Job drawing, mm, ordinate dimensions from the low corner. One solid piece. Give positions to 0.01 mm unless a question says otherwise; leave off trailing zeros. Order: outer loops, then holes, each group sorted by start corner. A loop starts at its lowest first (then second) coordinate and runs counter-clockwise, first axis right, second up. Notation, with made-up numbers: (7.5, 33.5) - (64.5, 33.5) arc R30 ccw to (64.5, 68.5) - close; hole circle Ø4 at (75.5, 39.25). An arc over 180 degrees is marked (long way). Write each question's results on one line, items separated by ' | '. Start each with the question number.
1) Cut at A-A on z = 301.5. List the corners of the cut face in (x, y).
2) Drop flat-ended pins along their axis: pin 1 Ø5 at (x, y) = (211, 175.5) entering from +Z (1 decimal); pin 2 Ø6 at (x, y) = (96, 358.5) entering from +Z; pin 3 Ø10 at (x, y) = (312.5, 371.5) entering from +Z. Give the stop position or say it passes through.
3) Cut at C-C on y = 450.5. List the corners of the cut face in (x, z), plus the area to 3 significant figures.
4) Drill centre lines: line 1 along X through (y, z) = (59, 75); line 2 along Y through (x, z) = (479, 47); line 3 along Z through (x, y) = (347, 65). Where is each one in solid material? Low to high. Write a range as from..to.
5) Cut at B-B on x = 260. List the corners of the cut face in (y, z) (1 decimal), plus the area to 3 significant figures.
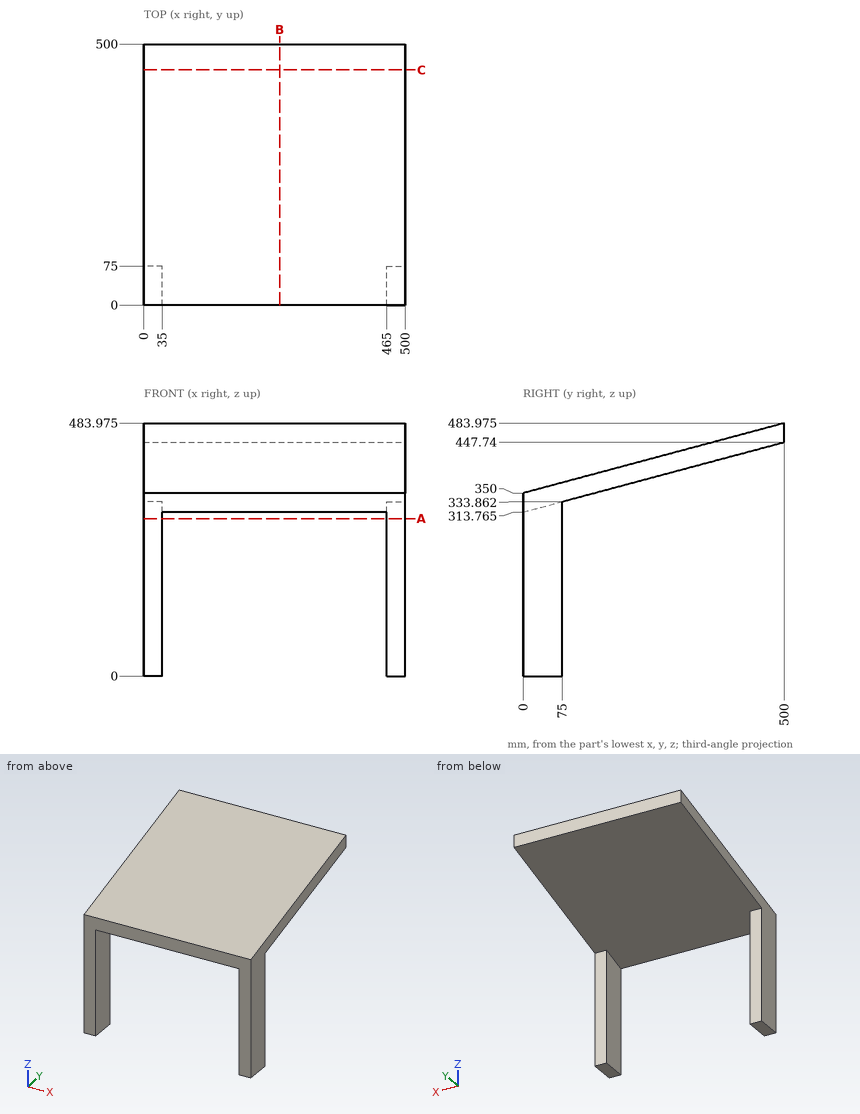
Results:
1) outline: (0, 0) - (35, 0) - (35, 75) - (0, 75) - close; (465, 0) - (500, 0) - (500, 75) - (465, 75) - close
2) pin 1: z = 397.7 | pin 2: z = 446.86 | pin 3: z = 450.88
3) outline: (0, 434.48) - (500, 434.48) - (500, 470.71) - (0, 470.71) - close | area: 18,100 mm^2
4) line 1: 0..35, 465..500 | line 2: 0..75 | line 3: 331.18..367.42
5) outline: (0, 313.8) - (500, 447.7) - (500, 484) - (0, 350) - close | area: 18,100 mm^2
